```python
from build123d import *

# Parameters (mm, degrees)
SKETCH1_W           = 31.75
SKETCH1_H           = 3.175
SKETCH1_W_2         = 3.175
SKETCH1_H_2         = 31.75
BOSS_EXTRUDE1_DEPTH = 3.175


with BuildPart() as part:
    # Sketch1 → Boss-Extrude1 (new body)
    with BuildSketch(Plane.XY):
        Polygon((-50.8, 28.575), (-44.45, 28.575), (-44.45, 32.385), (-38.1, 32.385), (-38.1, 28.575), (-34.925, 28.575), (-34.925, -19.05), (34.925, -19.05), (34.925, 28.575), (38.1, 28.575), (38.1, 32.385), (44.45, 32.385), (44.45, 28.575), (50.8, 28.575), (50.8, -34.29), (-50.8, -34.29), align=None)
        with Locations((0, -30.1625)):
            Rectangle(SKETCH1_W, SKETCH1_H, mode=Mode.SUBTRACT)
        with Locations((-46.0375, 0)):
            Rectangle(SKETCH1_W_2, SKETCH1_H_2, mode=Mode.SUBTRACT)
        with Locations((46.0375, 0)):
            Rectangle(SKETCH1_W_2, SKETCH1_H_2, mode=Mode.SUBTRACT)
    extrude(amount=BOSS_EXTRUDE1_DEPTH)


solid = part.part
```
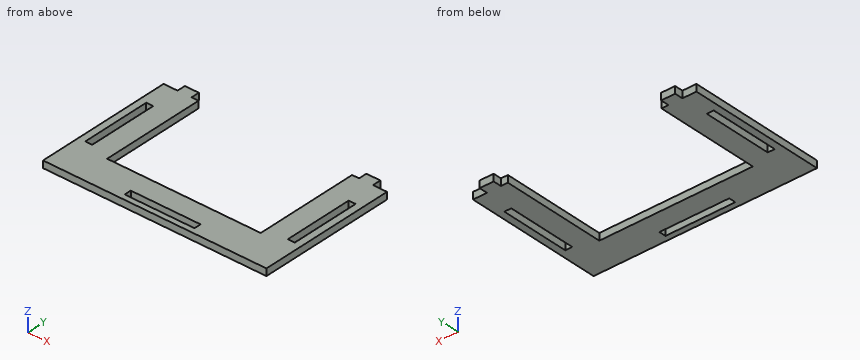
Verification items for the finished model (mm, model axes). Round coordinates to 2 decimals unless told otherwise and drop trailing zeros. Order: outer loops, then holes, each group sorted by start corner. A loop starts at its lowest first (then second) coordinate and runs counter-clockwise, first axis right, second up. Notation, with made-up numbers: (63.5, 77.25) -> (116.5, 77.25) arc R12 cw to (116.5, 90.25) -> close; hole circle Ø9 at (70.5, 64.5). An arc over 180 degrees is marked (long way). Put each result on its own line as item: value. Start each with the question number.
(1) Section check C-C (y = 18.5). Enter the section's corners in (x, z) (3 decimals), then the cut area to 3 significant figures.
(2) Section check A-A (y = 6). Enter the section's corners in (x, z) (3 decimals), then the cut area to 3 significant figures.
(3) Section check D-D (z = 0.75). Enter the section's corners in (x, y) (3 decimals).
(4) Section check B-B (x = -13). Enter the section's corners in (y, z) (3 decimals).
(5) Depth check by flat-ended pin: pin 1 Ø1 at (y, z) = (30, 2) entering from -X; pin 2 Ø1.6 at (y, z) = (31, 1) entering from +X; pin 3 Ø1.5 at (x, z) = (4, 1) entering from +Y. Enter the tip coordinate at first touch or a pass-through.
(6) Material ranges on line 1 along X through (y, z) = (13.5, 2.7) (3 decimals); line 2 along Y through (x, z) = (14, 1.3) (3 decimals); line 3 along X through (y, z) = (29.5, 1.4), recorded low to high.
Completed:
1. outline: (-50.8, 0) -> (-34.925, 0) -> (-34.925, 3.175) -> (-50.8, 3.175) -> close; (34.925, 0) -> (50.8, 0) -> (50.8, 3.175) -> (34.925, 3.175) -> close
1. area: 101 mm2
2. outline: (-50.8, 0) -> (-47.625, 0) -> (-47.625, 3.175) -> (-50.8, 3.175) -> close; (-44.45, 0) -> (-34.925, 0) -> (-34.925, 3.175) -> (-44.45, 3.175) -> close; (34.925, 0) -> (44.45, 0) -> (44.45, 3.175) -> (34.925, 3.175) -> close; (47.625, 0) -> (50.8, 0) -> (50.8, 3.175) -> (47.625, 3.175) -> close
2. area: 80.6 mm2
3. outline: (-50.8, -34.29) -> (50.8, -34.29) -> (50.8, 28.575) -> (44.45, 28.575) -> (44.45, 32.385) -> (38.1, 32.385) -> (38.1, 28.575) -> (34.925, 28.575) -> (34.925, -19.05) -> (-34.925, -19.05) -> (-34.925, 28.575) -> (-38.1, 28.575) -> (-38.1, 32.385) -> (-44.45, 32.385) -> (-44.45, 28.575) -> (-50.8, 28.575) -> close; hole (-47.625, -15.875) -> (-44.45, -15.875) -> (-44.45, 15.875) -> (-47.625, 15.875) -> close; hole (-15.875, -31.75) -> (15.875, -31.75) -> (15.875, -28.575) -> (-15.875, -28.575) -> close; hole (44.45, -15.875) -> (47.625, -15.875) -> (47.625, 15.875) -> (44.45, 15.875) -> close
4. outline: (-34.29, 0) -> (-31.75, 0) -> (-31.75, 3.175) -> (-34.29, 3.175) -> close; (-28.575, 0) -> (-19.05, 0) -> (-19.05, 3.175) -> (-28.575, 3.175) -> close
5. pin 1: stops at x = -44.45
5. pin 2: stops at x = 44.45
5. pin 3: stops at y = -19.05
6. line 1: x = -50.8 to -47.625, -44.45 to -34.925, 34.925 to 44.45, 47.625 to 50.8
6. line 2: y = -34.29 to -31.75, -28.575 to -19.05
6. line 3: x = -44.45 to -38.1, 38.1 to 44.45
